```python
from build123d import *

# Parameters (mm, degrees)
SKETCH1_R           = 19
SKETCH1_R_2         = 13.5
BOSS_EXTRUDE1_DEPTH = 26
SKETCH2_W           = 26
SKETCH2_H           = 0.5
SKETCH4_R           = 5
CUT_EXTRUDE1_DEPTH  = 10
SKETCH5_R           = 1.25
CUT_EXTRUDE4_DEPTH  = 20
SKETCH6_R           = 3
CUT_EXTRUDE5_DEPTH  = 20


with BuildPart() as part:
    # Sketch1 → Boss-Extrude1 (new body)
    with BuildSketch(Plane.XY):
        with Locations(Location((0, 0, 0), (0, 0, 180))):
            Circle(SKETCH1_R)
        with Locations(Location((0, 0, 0), (0, 0, 180))):
            Circle(SKETCH1_R_2, mode=Mode.SUBTRACT)
    extrude(amount=BOSS_EXTRUDE1_DEPTH)

    # Sketch2 → Cut-Revolve1 (revolve, cut)
    with BuildSketch(Plane(origin=(0, 0, 0), x_dir=(0, 0, -1), z_dir=(1, 0, 0)), mode=Mode.PRIVATE) as cut_revolve1_sk:
        with Locations((-13, 18.75)):
            Rectangle(SKETCH2_W, SKETCH2_H)
    revolve(cut_revolve1_sk.sketch.rotate(Axis((0, 0, 0), (0, 0, 1)), 90), axis=Axis((0, 0, 0), (0, 0, 1)), mode=Mode.SUBTRACT)

    # Sketch3 → Cut-Revolve2 (revolve, cut)
    with BuildSketch(Plane(origin=(0, 0, 0), x_dir=(0, 0, -1), z_dir=(1, 0, 0)), mode=Mode.PRIVATE) as cut_revolve2_sk:
        Polygon((0, 18), (0, 0), (-26, 0), (-26, 18), (-25, 18), (-25, 16.5), (-16, 16.5), (-16, 15.5), (-14, 15.5), (-14, 16.5), (-1, 16.5), (-1, 18), align=None)
    revolve(cut_revolve2_sk.sketch.rotate(Axis((0, 0, 26), (0, 0, -1)), 90), axis=Axis((0, 0, 26), (0, 0, -1)), mode=Mode.SUBTRACT)

    # Sketch4 → Cut-Extrude1 (cut)
    with BuildSketch(Plane(origin=(9.25, 16.02146997, 0), x_dir=(-0.866025403784438, 0.500000000000001, 0), z_dir=(0.500000000000001, 0.866025403784438, 0))):
        with Locations((0, 7.7)):
            Circle(SKETCH4_R)
    cut_extrude1 = extrude(amount=-CUT_EXTRUDE1_DEPTH, mode=Mode.SUBTRACT)

    # Mirror1: Cut-Extrude1 across plane
    add(cut_extrude1.mirror(Plane(origin=(0, 0, 0), x_dir=(0, 0, 1), z_dir=(1, 0, 0))), mode=Mode.SUBTRACT)

    # Sketch5 → Cut-Extrude4 (cut)
    with BuildSketch(Plane(origin=(0, 0, 0), x_dir=(1, 0, 0), z_dir=(0, 1, 0))):
        with Locations(Location((0, -15, 0), (0, 0, 270))):
            Circle(SKETCH5_R)
    extrude(amount=-CUT_EXTRUDE4_DEPTH, mode=Mode.SUBTRACT)

    # Sketch6 → Cut-Extrude5 (cut)
    with BuildSketch(Plane(origin=(0, 0, 0), x_dir=(0, 0, -1), z_dir=(1, 0, 0))):
        with Locations((-20, 0)):
            Circle(SKETCH6_R)
    extrude(amount=-CUT_EXTRUDE5_DEPTH, mode=Mode.SUBTRACT)


solid = part.part
```
Geometry: final body of the model. Coordinates: model frame, mm. A direction names the side the tool comes from. Coordinates: 2 decimals unless noted, no trailing zeros. Order: outer loops, then holes, each group sorted by start corner. A loop starts at its lowest first (then second) coordinate and runs counter-clockwise, first axis right, second up.
Item 1: Section query A-A (x = 0). Output: boundary loops of the cut face in (y, z).
Answer:
outline: (-18.5, 0) - (-18, 0) - (-18, 1) - (-16.5, 1) - (-16.5, 13.75) - (-18.5, 13.75) - close; (-18.5, 16.25) - (-16.5, 16.25) - (-16.5, 25) - (-18, 25) - (-18, 26) - (-18.5, 26) - close; (15.5, 14) - (16.5, 14) - (16.5, 1) - (18, 1) - (18, 0) - (18.5, 0) - (18.5, 26) - (18, 26) - (18, 25) - (16.5, 25) - (16.5, 16) - (15.5, 16) - close
Item 2: Contact query for flat-ended pins moving along their axis: P1, Ø1.5, axis at x = 0, z = 15, coming from the -Y side; P2, Ø8, axis at y = -12.5, z = 5, coming from the +X side; P3, Ø10, axis at y = -9.5, z = 4.5, coming from the +X side; P4, Ø8, axis at y = 0, z = 20, coming from the -X side. Output: stop coordinate, or through.
Answer:
P1: stops at y = 15.48
P2: stops at x = 16.43
P3: stops at x = 17.94
P4: stops at x = -18.5
Item 3: Access query for faces 1 (the face through (0.05, -16.95, 13.75)), 2 (the face through (-17, 0, 23)), 3 (the face through (15.738, -4.956, 20.437)), 4 (the face through (-13.267, -12.165, 0.493)). Directions: +Z, -Z, +X, -X, +Y, -Y. A direction counts if a zero-diameter tool reaches every point of the face in a straight line with its end or side. Return the directions, or none.
Answer:
face 1: -Y
face 2: -X
face 3: +Z
face 4: -Z
Item 4: Draft query along Y for faces 5 (the face through (-15, 5, 16)), 6 (the face through (13.64, -12.5, 12.82)), 7 (the face through (-4.02, 17.73, 26)). Return one class per face: released by +Y, released by -Y, zero draft, split by the parting line, or undercut.
Answer:
face 5: undercut
face 6: split by the parting line
face 7: zero draft
Item 5: Section query C-C (y = -13). Output: boundary loops of the cut face in (x, z), then the cut area to 3 significant figures.
Answer:
outline: (-13.16, 0) - (-12.45, 0) - (-12.45, 1) - (-10.16, 1) - (-10.16, 14) - (-8.44, 14) - (-8.44, 16) - (-10.16, 16) - (-10.16, 25) - (-12.45, 25) - (-12.45, 26) - (-13.16, 26) - close; (8.44, 14) - (10.16, 14) - (10.16, 1) - (12.45, 1) - (12.45, 0) - (13.16, 0) - (13.16, 26) - (12.45, 26) - (12.45, 25) - (10.16, 25) - (10.16, 16) - (8.44, 16) - close
area: 154 mm2
Item 6: Section query B-B (y = 2.5). Output: boundary loops of the cut face in (x, z), then the cut area to 3 significant figures.
Answer:
outline: (-18.33, 0) - (-17.83, 0) - (-17.83, 1) - (-16.31, 1) - (-16.31, 14) - (-15.3, 14) - (-15.3, 16) - (-16.31, 16) - (-16.31, 18.34) - (-18.33, 18.34) - close; (-18.33, 21.66) - (-16.31, 21.66) - (-16.31, 25) - (-17.83, 25) - (-17.83, 26) - (-18.33, 26) - close; (15.3, 14) - (16.31, 14) - (16.31, 1) - (17.83, 1) - (17.83, 0) - (18.33, 0) - (18.33, 26) - (17.83, 26) - (17.83, 25) - (16.31, 25) - (16.31, 16) - (15.3, 16) - close
area: 96.4 mm2
Item 7: Section query D-D (z = 24). Output: boundary loops of the cut face in (x, y).
Answer:
outline: circle Ø37 at (0, 0); hole circle Ø33 at (0, 0)
Item 8: Material intervals for line 1 along Z through (x, y) = (-5, 15.5); line 2 along Y through (x, z) = (-12.5, 5); line 3 along Z through (x, y) = (-15.5, 8), sorted ascending.
Answer:
line 1: z = 14 to 16
line 2: y = -13.64 to -10.77, 10.77 to 13.23
line 3: z = 1 to 25
